Design review of the part built by this model. Coordinates are the model's own, in mm. A direction names the side the tool comes from. Coordinates: 2 decimals unless noted, no trailing zeros. Order: outer loops, then holes, each group sorted by start corner. A loop starts at its lowest first (then second) coordinate and runs counter-clockwise, first axis right, second up. Notation, with made-up numbers: M 41,82.5 L 94,82.5 A17 cw 94,113.5 Z; hole C 27.5,84.25 d10. An arc over 180 degrees is marked long. Use CSV: the item, a comma, the result in double quotes.
```python
from build123d import *

# Parameters (mm, degrees)
F0_W     = 1600.2
F0_H     = 762
F1_DEPTH = 304.8
F2_T     = -12.7
F3_W     = 12.7
F3_H     = 736.6
F4_DEPTH = 292.1


with BuildPart() as f1:
    # F0 (on Front) → F1 (new body)
    with BuildSketch(Plane.XZ):
        Rectangle(F0_W, F0_H)
    extrude(amount=-F1_DEPTH)

    # F2
    f2_openings = [f1.faces().sort_by_distance(p)[0] for p in [
        (0, 0, 0),
    ]]
    offset(amount=F2_T, openings=f2_openings)

    # F3 (on face) → F4 (join)
    with BuildSketch(Plane.XZ.offset(-292.1)):
        with Locations((-228.6, 0)):
            Rectangle(F3_W, F3_H)
        with Locations((228.6, 0)):
            Rectangle(F3_W, F3_H)
    extrude(amount=F4_DEPTH)


solid = f1.part
```
(1) The part is to be moulded in two halves that separate along X. For faces 3 (the face through (-11, 150, 381)), 4 (the face through (-800.1, 150, -5)), 5 (the face through (234.95, 148, -5)), say which applies: pulls with the +X half, pulls with the -X half, needs draft (parallel to the pull), parting line crosses it, or undercut.
The answers:
face 3,"needs draft"
face 4,"pulls with the -X half"
face 5,"undercut"
(2) Add section A-A on y = 146.5. State the section outline as (x, z) points, and give its area (3 significant figures).
The answers:
outline,"M -800.1,-381 L 800.1,-381 L 800.1,381 L -800.1,381 Z; hole M -787.4,-368.3 L -234.95,-368.3 L -234.95,368.3 L -787.4,368.3 Z; hole M -222.25,-368.3 L 222.25,-368.3 L 222.25,368.3 L -222.25,368.3 Z; hole M 234.95,-368.3 L 787.4,-368.3 L 787.4,368.3 L 234.95,368.3 Z"
area,"78,100 mm2"
(3) For faces 1 (the face through (233, 0, 171)), 2 (the face through (-234.95, 148, -5)), list the 3-axis set-ups (+Z, -Z, +X, -X, +Y, -Y) from which the entire face can be reached by the end or side of a thin tool; tool diameter is ignored.
The answers:
face 1,"+Z, -Z, +X, -X, -Y"
face 2,"-Y"
(4) Add section B-B on z = 41. State the section outline as (x, y) points, and give its area (3 significant figures).
The answers:
outline,"M -800.1,0 L -787.4,0 L -787.4,292.1 L -234.95,292.1 L -234.95,0 L -222.25,0 L -222.25,292.1 L 222.25,292.1 L 222.25,0 L 234.95,0 L 234.95,292.1 L 787.4,292.1 L 787.4,0 L 800.1,0 L 800.1,304.8 L -800.1,304.8 Z"
area,"35,200 mm2"
(5) Wall thickness on probe 1 along X at (y, z) = (242, -44); probe 2 along Z at (x, y) = (196.5, 48); probe 3 along Y at (x, z) = (-715, -332.5): over which ranges is each line inside the solid? List them lowest first.
The answers:
probe 1,"x = -800.1 to -787.4, -234.95 to -222.25, 222.25 to 234.95, 787.4 to 800.1"
probe 2,"z = -381 to -368.3, 368.3 to 381"
probe 3,"y = 292.1 to 304.8"
(6) Add section C-C on x = 290. State the section outline as (y, z) points, and give its area (3 significant figures).
The answers:
outline,"M 0,-381 L 304.8,-381 L 304.8,381 L 0,381 L 0,368.3 L 292.1,368.3 L 292.1,-368.3 L 0,-368.3 Z"
area,"17,100 mm2"
